Verification items for this drawing (mm, ordinates from the low corner). Give positions to 0.01 mm unless a question says otherwise; leave off trailing zeros. Order: outer loops, then holes, each group sorted by start corner. A loop starts at its lowest first (then second) coordinate and runs counter-clockwise, first axis right, second up. Notation, with made-up numbers: (79.25, 64) -> (98.25, 64) arc R22 ccw to (98.25, 77) -> close; hole circle Ø6 at (-35, -38.75). An arc over 180 degrees is marked (long way). One line per question, with ' | ' between items.
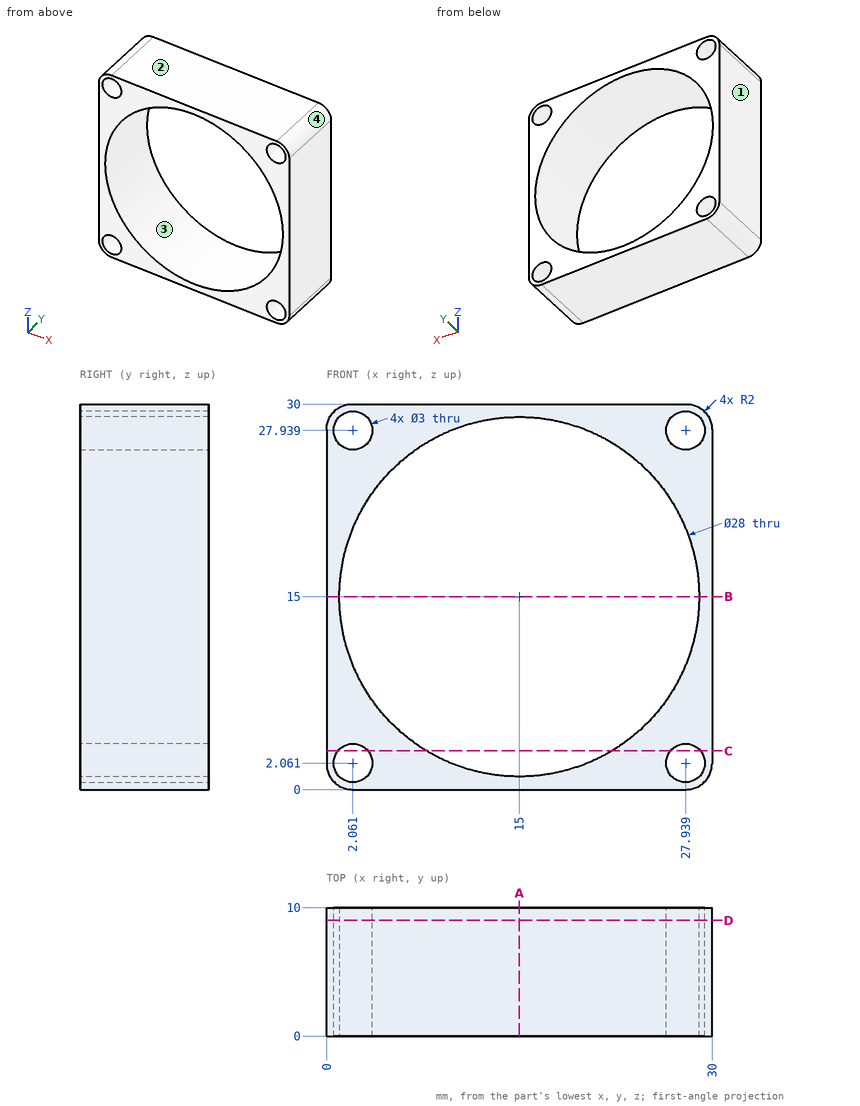
Q1. Section check D-D (y = 9). Enter the section's corners in (x, z).
Result sheet:
outline: (0, 2) arc R2 ccw to (2, 0) -> (28, 0) arc R2 ccw to (30, 2) -> (30, 28) arc R2 ccw to (28, 30) -> (2, 30) arc R2 ccw to (0, 28) -> close; hole circle Ø3 at (2.06, 2.06); hole circle Ø3 at (2.06, 27.94); hole circle Ø28 at (15, 15); hole circle Ø3 at (27.94, 2.06); hole circle Ø3 at (27.94, 27.94)
Q2. Thickness scan on line 1 (Z direction, x = 14.75, y = 5.75); line 2 (X direction, y = 3.25, z = 28) (1 decimal). Record the ranges inside material, lowest first.
Result sheet:
line 1: z = 0 to 1, 29 to 30 | line 2: x = 0 to 0.6, 3.6 to 9.8, 20.2 to 26.4, 29.4 to 30
Q3. Mould release check, pull along X, two halves, no side actions. Record for the marked faces 1, 2, 3 and 4: pulls with the +X half, pulls with the -X half, needs draft (parallel to the pull), parting line crosses it, or undercut.
Result sheet:
face 1: pulls with the -X half | face 2: needs draft | face 3: undercut | face 4: pulls with the +X half
Q4. Section check B-B (z = 15). Enter the section's corners in (x, y), and give its area (3 significant figures).
Result sheet:
outline: (0, 0) -> (1, 0) -> (1, 10) -> (0, 10) -> close; (29, 0) -> (30, 0) -> (30, 10) -> (29, 10) -> close | area: 20.0 mm2
Q5. Section check A-A (x = 15). Enter the section's corners in (y, z), and give its area (3 significant figures).
Result sheet:
outline: (0, 0) -> (10, 0) -> (10, 1) -> (0, 1) -> close; (0, 29) -> (10, 29) -> (10, 30) -> (0, 30) -> close | area: 20.0 mm2
Q6. Section check C-C (z = 3). Enter the section's corners in (x, y), and give its area (3 significant figures).
Result sheet:
outline: (0, 0) -> (0.89, 0) -> (0.89, 10) -> (0, 10) -> close; (3.23, 0) -> (7.79, 0) -> (7.79, 10) -> (3.23, 10) -> close; (22.21, 0) -> (26.77, 0) -> (26.77, 10) -> (22.21, 10) -> close; (29.11, 0) -> (30, 0) -> (30, 10) -> (29.11, 10) -> close | area: 109 mm2
